Check sheet for the modelled part. Datum: model origin and axes. Units: mm. A direction names the side the tool comes from. Round coordinates to 2 decimals unless told otherwise and drop trailing zeros. Order: outer loops, then holes, each group sorted by start corner. A loop starts at its lowest first (then second) coordinate and runs counter-clockwise, first axis right, second up.
Q1. Scan lines: probe 1 along Z at (x, y) = (-67, 3); probe 2 along X at (y, z) = (13.5, -86.5); probe 3 along X at (y, z) = (31, -30). Record each from-to range of solid material in increasing order.
Q2. Set-up check for faces 4 (the cylindrical face through (-59.72, 7.51, -67.17)), 5 (the cylindrical face through (-16.1, 5.4, -92.69)), 6 (the cylindrical face through (-35.738, 27.49, -123.845)): record each of +Z, -Z, +X, -X, +Y, -Y from which the full face is reachable in a straight line by a thin tool's end or side.
Q3. Cross-section at B-B on x = -11. Record the cut outline in (y, z) (3 decimals), then the cut area to 3 significant figures.
Q4. Cross-section at C-C on z = -104.5. Record the cut outline in (x, y), then the cut area to 3 significant figures.
Q5. Mould release check, pull along X, two halves, no side actions. Record for faces 1 (the flat face through (-42, 21, 0)), 2 (the conical face through (-33.326, 6.897, -89.588)), 3 (the flat face through (-68, 12.7, -115)): +X half, -X half, draft (parallel to the pull), parting line (faces both ways), or undercut.
Q6. Depth check by flat-ended pin: P1, Ø1.9, axis at y = 6.55, z = -65.91, coming from the -X side; P2, Ø11.5, axis at x = -69.5, z = -9, coming from the +Y side; P3, Ø5.5, axis at y = 6.35, z = -89.66, coming from the +X side. Enter the tip coordinate at first touch or a pass-through.
Q7. Cross-section at A-A on y = 21.5. Give the number of separate pieces and of enclosed holes in the cut face, then the cut area to 3 significant figures.
Autodesk Inventor part; units mm, degrees
ref_plane "YZ Plane" through (0, 0, 0) normal (1, 0, 0) x (0, 1, 0)
ref_plane "XZ Plane" through (0, 0, 0) normal (0, 1, 0) x (-1, 0, 0)
ref_plane "XY Plane" through (0, 0, 0) normal (0, 0, 1) x (1, 0, 0)
sketch "Sketch1" plane through (0, 0, 0) normal (0, 1, 0) x (-1, 0, 0)
  line L0 (0, 0) -> (85.48, 0)
  line L1 (85.48, 0) -> (85.48, -127.76)
  line L2 (85.48, -127.76) -> (0, -127.76)
  line L3 (0, -127.76) -> (0, 0)
  line L4 (85.48, 0) -> (67.5195, -17.9605)
  line L5 (85.48, 0) -> (110.88, 0) construction
  line L6 (0, 0) -> (17.9605, -17.9605)
  line L7 (85.48, -127.76) -> (67.5195, -109.7995)
  line L8 (85.48, -127.76) -> (110.88, -127.76) construction
  line L9 (0, -127.76) -> (17.9605, -109.7995)
  line L10 (0, -127.76) -> (25.4, -127.76) construction
  dimension "d0" = 85.48
  dimension "d1" = 127.76
  dimension "d2" = 25.4
  dimension "d3" = 135
  dimension "d4" = 25.4
  dimension "d5" = 25.4
  dimension "d6" = 135
  dimension "d7" = 25.4
  dimension "d8" = 45
extrude "Extrusion1" add sketch "Sketch1" along normal blind 42.7
sketch "Sketch2" plane through (0, 0, 0) normal (0, -1, 0) x (1, 0, 0)
  line L0 (-85.48, 0) -> (0, 0)
  line L1 (0, 0) -> (-17.9605, -17.9605)
  line L2 (0, 0) -> (25.4, 0) construction
  line L3 (0, 0) -> (0, -127.76)
  line L4 (0, -127.76) -> (-17.9605, -109.7995)
  line L5 (0, -127.76) -> (25.4, -127.76) construction
  line L6 (-85.48, -127.76) -> (-85.48, 0)
  line L7 (-85.48, 0) -> (-67.5195, -17.9605)
  line L8 (-85.48, 0) -> (-60.08, 0) construction
  line L9 (0, -127.76) -> (-85.48, -127.76)
  line L10 (-85.48, -127.76) -> (-67.5195, -109.7995)
  line L11 (-85.48, -127.76) -> (-60.08, -127.76) construction
  dimension "d11" = 25.4
  dimension "d12" = 135
  dimension "d13" = 25.4
  dimension "d14" = 135
  dimension "d15" = 25.4
  dimension "d16" = 45
  dimension "d17" = 25.4
  dimension "d18" = 45
hole "Hole1" at (-17.9605, 0, -17.9605) at (-67.5195, 0, -17.9605) at (-67.5195, 0, -109.7995) at (-17.9605, 0, -109.7995) direction (0, 1, 0) diameter 3.683 depth 9.525 tip angle 118
sketch "Sketch4" plane through (0, 42.7, 0) normal (0, 1, 0) x (1, 0, 0)
  line L0 (0, -1.0521) -> (19.05, -1.0521) construction
  line L1 (0, 0) -> (0, 127.76)
  line L2 (0, 18.3507) -> (0, 0)
  line L3 (0, 0) -> (-18.7946, 0)
  line L4 (0, 0) -> (-17.3355, 0)
  line L5 (-17.3355, 0) -> (-17.3355, 13.1191)
  line L6 (-17.3355, 13.1191) -> (0, 13.1191)
  line L7 (0, 13.1191) -> (0, 0)
  dimension "d41" = 17.3355
  dimension "d42" = 13.1191
hole "Hole2" at (-17.3355, 42.7, -13.1191) direction (0, -1, 0) diameter 23 depth 30
pattern_linear "Rectangular Pattern1" count 3 spacing 25.4 along (-1, 0, 0) count 5 spacing 25.4 along (0, 0, -1) of "Hole2"
sketch "Sketch5" plane through (-85.48, 0, -127.76) normal (-1, 0, 0) x (0, 0, 1)
  line L0 (127.76, 0) -> (127.76, 42.7)
  line L1 (127.76, 0) -> (89.66, 0)
  line L2 (89.66, 0) -> (89.66, 6.35)
  line L3 (89.66, 6.35) -> (127.76, 6.35)
  line L4 (127.76, 6.35) -> (127.76, 0)
  line L5 (62.646, 6.35) -> (127.76, 6.35)
  line L6 (127.76, 6.35) -> (127.76, 0)
  line L7 (127.76, 0) -> (62.646, 0)
  line L8 (62.646, 0) -> (62.646, 6.35)
  dimension "d43" = 38.1
  dimension "d44" = 6.35
hole "Hole3" at (-85.48, 6.35, -38.1) direction (1, 0, 0) diameter 6.35 depth 31.75 tip angle 118
sketch "Sketch6" plane through (-85.48, 0, -127.76) normal (-1, 0, 0) x (0, 0, 1)
  line L0 (61.854, 6.5465) -> (127.76, 6.5465)
  line L1 (127.76, 6.5465) -> (127.76, 0.1965)
  line L2 (127.76, 0.1965) -> (61.854, 0.1965)
  line L3 (61.854, 0.1965) -> (61.854, 6.5465)
  point P0 (127.76, 0)
  dimension "d52" = 6.35
hole "Hole4" at (-85.48, 6.5465, -65.906) direction (1, 0, 0) diameter 3.175 depth 50.8 tip angle 118
sketch "Sketch7" plane through (0, 0, 0) normal (1, 0, 0) x (0, 0, -1)
  line L0 (127.76, 0) -> (0, 0)
  line L1 (127.76, 0) -> (89.66, 0)
  line L2 (89.66, 0) -> (89.66, 6.35)
  line L3 (89.66, 6.35) -> (127.76, 6.35)
  line L4 (127.76, 6.35) -> (127.76, 0)
  dimension "d60" = 38.1
  dimension "d61" = 6.35
hole "Hole5" at (0, 6.35, -89.66) direction (-1, 0, 0) diameter 6.35 depth 31.75 tip angle 118
properties part number "Thermal_topplate_8mL"
Results found:
1. probe 1: z = -127.76 to -111.57, -108.03 to -19.73, -16.19 to 0
1. probe 2: x = -85.48 to -79.28, -56.99 to -53.88, -31.59 to -28.48, -6.19 to 0
1. probe 3: x = -85.48 to -75.86, -60.41 to -50.46, -35.01 to -25.06, -9.61 to 0
2. face 4: -X
2. face 5: +X
2. face 6: +Y
3. outline: (0, -127.76) - (42.7, -127.76) - (42.7, -124.317) - (12.7, -124.317) - (12.7, -105.122) - (42.7, -105.122) - (42.7, -98.917) - (12.7, -98.917) - (12.7, -79.722) - (42.7, -79.722) - (42.7, -73.517) - (12.7, -73.517) - (12.7, -54.322) - (42.7, -54.322) - (42.7, -48.117) - (12.7, -48.117) - (12.7, -28.922) - (42.7, -28.922) - (42.7, -22.717) - (12.7, -22.717) - (12.7, -3.522) - (42.7, -3.522) - (42.7, 0) - (0, 0) - close; hole circle Ø6.35 at (6.35, -89.66)
3. area: 2,540 mm2
4. outline: (-85.48, 0) - (0, 0) - (0, 42.7) - (-12.06, 42.7) - (-12.06, 12.7) - (-22.61, 12.7) - (-22.61, 42.7) - (-37.46, 42.7) - (-37.46, 12.7) - (-48.01, 12.7) - (-48.01, 42.7) - (-62.86, 42.7) - (-62.86, 12.7) - (-73.41, 12.7) - (-73.41, 42.7) - (-85.48, 42.7) - close
4. area: 2,700 mm2
5. face 1: draft
5. face 2: +X half
5. face 3: undercut
6. P1: stops at x = -34.3
6. P2: stops at y = 12.7
6. P3: stops at x = -32.01
7. separate pieces: 1
7. enclosed holes: 15
7. area: 4,690 mm2
